from build123d import *

# Parameters (mm, degrees)
F1_DEPTH    = 8
F2_R        = 1
F3_T1_DEPTH = 64.2226111809
F3_T3_DEPTH = 65.5041643561
F3_T5_DEPTH = 66.9229315715
F3_T7_DEPTH = 64.2892221554
F3_T9_DEPTH = 66.1623607225


# Not quite as in the source:
# - a fillet or chamfer that OpenCascade refuses, or shapes differently, is made with other operations: its cross-section is extruded or revolved along the edge and cut away or added


with BuildPart() as f1:
    # F0 (on Top) → F1 (new body)
    with BuildSketch(Plane.XY):
        with BuildLine():
            ThreePointArc((1.7213359453, 34.45703125), (0, 29), (-1.7213359453, 34.45703125))
            ThreePointArc((-1.7213359453, 34.45703125), (-5.6630518779, 34.0320414232), (-9.5299848811, 33.1576444906))
            ThreePointArc((-9.5299848811, 33.1576444906), (-4.4795318248, 25.2311781209), (-2.7128129211, 16))
            ThreePointArc((-2.7128129211, 16), (-12.2077903389, -3.6110753077), (-33.4803548991, -8.3256132406))
            ThreePointArc((-33.4803548991, -8.3256132406), (-32.3848639744, -11.8941407997), (-30.9102371196, -15.3234213285))
            ThreePointArc((-30.9102371196, -15.3234213285), (-25.3652162283, -14.4450583373), (-28.9498248331, -18.7658637459))
            ThreePointArc((-28.9498248331, -18.7658637459), (-26.6234342426, -21.9418036891), (-23.950370018, -24.83203125))
            ThreePointArc((-23.950370018, -24.83203125), (0, -7), (23.950370018, -24.83203125))
            ThreePointArc((23.950370018, -24.83203125), (26.587584538, -21.9852302339), (28.8884099574, -18.8602696198))
            ThreePointArc((28.8884099574, -18.8602696198), (24.9364218636, -14.6683482508), (30.5204410338, -16.0857912178))
            ThreePointArc((30.5204410338, -16.0857912178), (32.2347725379, -12.2950981871), (33.4803548991, -8.3256132406))
            ThreePointArc((33.4803548991, -8.3256132406), (6.0621778265, 3.5), (9.5299848811, 33.1576444906))
            ThreePointArc((9.5299848811, 33.1576444906), (5.6630518779, 34.0320414232), (1.7213359453, 34.45703125))
        make_face()
    extrude(amount=F1_DEPTH)

    # F2
    f2_edges = [f1.edges().sort_by_distance(p)[0] for p in [
        (-30.910237, -15.323421, 4),
        (-28.949825, -18.765864, 4),
        (1.721336, 34.457031, 4),
        (-1.721336, 34.457031, 4),
        (28.88841, -18.86027, 4),
        (30.520441, -16.085791, 4),
    ]]
    fillet(f2_edges, radius=F2_R)

    # F3: fillet of radius 20 on 6 edges, made by hand

    # F3_s2 → F3_t1 (cut)
    with BuildSketch(Plane.XY.offset(-28.1113055904)):
        with BuildLine():
            ThreePointArc((-22.2360329208, -8.3927218823), (-27.3415731158, -10.3001532277), (-31.7425915451, -13.5150982979))
            ThreePointArc((-31.7425915451, -13.5150982979), (-32.7145361346, -10.9548676622), (-33.4803548991, -8.3256132406))
            ThreePointArc((-33.4803548991, -8.3256132406), (-27.8620158848, -8.9995547655), (-22.2360329208, -8.3927218823))
        make_face()
    extrude(amount=F3_T1_DEPTH, mode=Mode.SUBTRACT)

    # F3_s4 → F3_t3 (cut)
    with BuildSketch(Plane.XY.offset(-28.7520821781)):
        with BuildLine():
            ThreePointArc((-3.9009970628, 34.2787430037), (-4.619010619, 28.731142286), (-3.7725584788, 23.2016815561))
            ThreePointArc((-3.7725584788, 23.2016815561), (-6.0709826163, 28.5152379545), (-9.5299848811, 33.1576444906))
            ThreePointArc((-9.5299848811, 33.1576444906), (-6.7388451877, 33.8354542682), (-3.9009970628, 34.2787430037))
        make_face()
        with BuildLine():
            ThreePointArc((3.9009970628, 34.2787430037), (4.619010619, 28.731142286), (3.7725584788, 23.2016815561))
            ThreePointArc((3.7725584788, 23.2016815561), (6.0709826163, 28.5152379545), (9.5299848811, 33.1576444906))
            ThreePointArc((9.5299848811, 33.1576444906), (6.7388451877, 33.8354542682), (3.9009970628, 34.2787430037))
        make_face()
    extrude(amount=F3_T3_DEPTH, mode=Mode.SUBTRACT)

    # F3_s6 → F3_t5 (cut)
    with BuildSketch(Plane.XY.offset(-29.4614657857)):
        with BuildLine():
            ThreePointArc((21.695923744, -8.2651405236), (27.0245333746, -10.4395796023), (31.513317936, -14.0413956808))
            ThreePointArc((31.513317936, -14.0413956808), (32.6222611015, -11.2266682781), (33.4803548991, -8.3256132406))
            ThreePointArc((33.4803548991, -8.3256132406), (27.5845251828, -8.999670843), (21.695923744, -8.2651405236))
        make_face()
    extrude(amount=F3_T5_DEPTH, mode=Mode.SUBTRACT)

    # F3_s8 → F3_t7 (cut)
    with BuildSketch(Plane.XY.offset(-28.1446110777)):
        with BuildLine():
            ThreePointArc((27.5839500196, -20.7213827076), (22.5899865116, -18.5199962805), (18.3770596718, -15.0505552356))
            ThreePointArc((18.3770596718, -15.0505552356), (21.7214673604, -19.6234958203), (23.950370018, -24.83203125))
            ThreePointArc((23.950370018, -24.83203125), (25.8490017853, -22.8490504552), (27.5839500196, -20.7213827076))
        make_face()
    extrude(amount=F3_T7_DEPTH, mode=Mode.SUBTRACT)

    # F3_s10 → F3_t9 (cut)
    with BuildSketch(Plane.XY.offset(-29.0811803612)):
        with BuildLine():
            ThreePointArc((-18.1139750308, -14.7696805432), (-22.5633062196, -18.281704114), (-27.8192704457, -20.4043669804))
            ThreePointArc((-27.8192704457, -20.4043669804), (-25.9793181426, -22.7007715474), (-23.950370018, -24.83203125))
            ThreePointArc((-23.950370018, -24.83203125), (-21.6255637275, -19.4566753424), (-18.1139750308, -14.7696805432))
        make_face()
    extrude(amount=F3_T9_DEPTH, mode=Mode.SUBTRACT)


solid = f1.part
Design review of the part built by this model. Coordinates are the model's own, in mm. A direction names the side the tool comes from. Round coordinates to 2 decimals unless told otherwise and drop trailing zeros. Loops run counter-clockwise (first coordinate to the right, second up) from the corner with the lowest first, then second, coordinate; pieces in that order, holes last. Notation, with made-up numbers: (86, -1) - (105, -1) arc R14 cw to (105, 16) - close; hole circle Ø11 at (-5.5, 87.5). An arc over 180 degrees is marked (long way). One line per item, written item: value. Start each with the question number.
1) Draft analysis for pull direction Y (two halves, no side actions). For faces 3 (the cylindrical face through (4.62, 28.81, 3.94)), 4 (the cylindrical face through (-27.27, -10.26, 3.94)), 5 (the cylindrical face through (0, -7, 4)), state which applies: +Y half, -Y half, draft (parallel to the pull), parting line (faces both ways), or undercut.
2) To check wall thickness, follow L1, parallel to Y at x = 26.5, z = 2.5; L2, parallel to X at y = -15, z = 4.5; L3, parallel to Y at x = 0, z = 5.25. State the ranges of each line that lie inside material, in increasing order. Write a range as from..to.
3) For faces 1 (the cylindrical face through (0, 29, 4)), 2 (the cylindrical face through (22.655, -18.56, 3.944)), list the 3-axis set-ups (+Z, -Z, +X, -X, +Y, -Y) from which the entire face can be reached by the end or side of a thin tool; tool diameter is ignored.
4) Consider section A-A on y = 32. Give the boundary of the cut face in (x, z).
5) Consider section B-B on x = 0. Give the boundary of the cut face in (y, z), then the cut area to 3 significant figures.
6) Consider section C-C on y = 22. Give the boundary of the cut face in (x, z), then the cut area to 3 significant figures.
7) Insertion check: pin 1 Ø3.5 at (x, y) = (0, 32) entering from +Z; pin 2 Ø3 at (x, z) = (17.5, 2) entering from +Y. Each pin has a flat end and moves straight along its axis. Give the tip position at first contact, or say it passes through.
Reported:
1. face 3: undercut
1. face 4: +Y half
1. face 5: -Y half
2. L1: y = -20.38..-19.01, -13.37..-10.14
2. L2: x = -25.12..-18.34, 18.33..24.77
2. L3: y = -7..29
3. face 1: +Z, -Z
3. face 2: +Z, -Z, -Y
4. outline: (-4.39, 0) - (-3, 0) - (-3, 8) - (-4.39, 8) - close; (3, 0) - (4.39, 0) - (4.39, 8) - (3, 8) - close
5. outline: (-7, 0) - (29, 0) - (29, 8) - (-7, 8) - close
5. area: 288 mm^2
6. outline: (-3.44, 0) - (3.44, 0) - (3.44, 8) - (-3.44, 8) - close
6. area: 55.1 mm^2
7. pin 1: passes through
7. pin 2: stops at y = -6.09
